The figure shows three views and two pictorial views of one solid part (mm, origin at its lowest corner). Answer the questions. Give positions to 0.01 mm unless a question says otherwise; leave off trailing zeros. Write each loop counter-clockwise with the first axis right and the second up, starting at its lowest first coordinate (ties: lowest second). Pieces come first, ordered by that corner, then holes. Notation, with made-up numbers: (1.5, 70) -> (60.5, 70) arc R30 ccw to (60.5, 102) -> close; hole circle Ø10 at (37.5, -28). An arc over 180 degrees is marked (long way). Use a Markdown table: item, result.
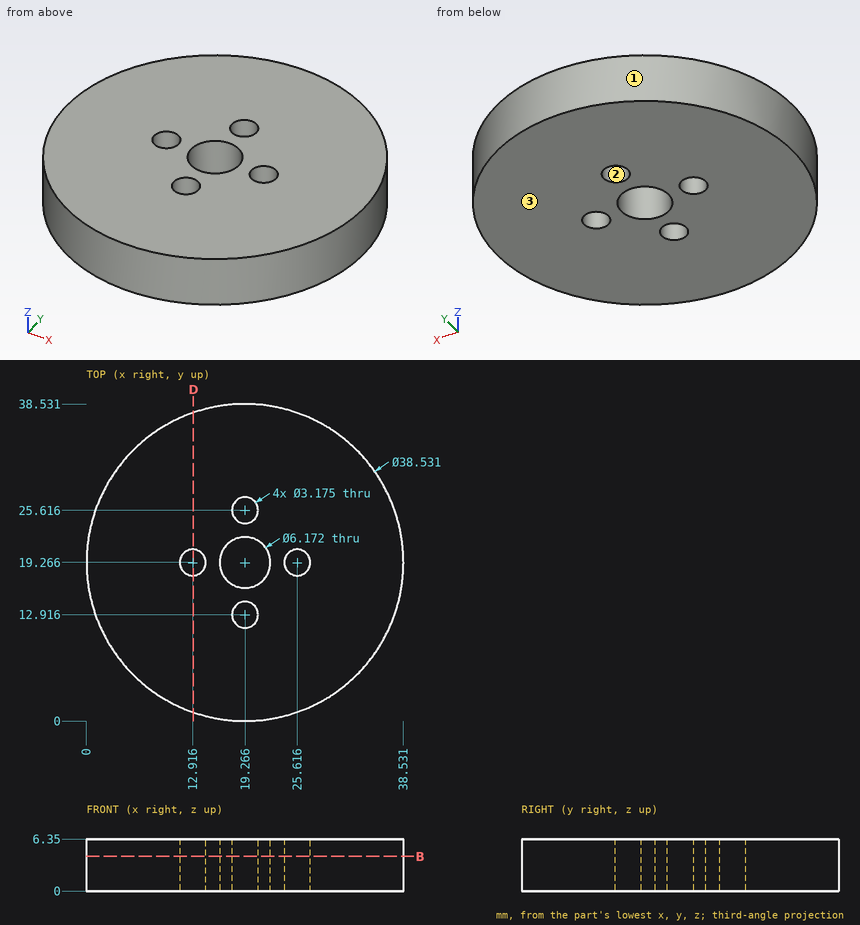
Item 1: A cutting plane is placed at D-D (x = 13). Give the vertices of the cut face in (y, z).
Return value:
| item | result |
|---|---|
| outline | (1.05, 0) -> (17.68, 0) -> (17.68, 6.35) -> (1.05, 6.35) -> close; (20.85, 0) -> (37.48, 0) -> (37.48, 6.35) -> (20.85, 6.35) -> close |
Item 2: Straight lines are drawn through the part: line 1 along X through (y, z) = (19.5, 5.5) (1 decimal); line 2 along X through (y, z) = (19, 1); line 3 along Y through (x, z) = (26, 2) (1 decimal). For each, find the intervals that lie inside material, in ascending order. Write a range as [from, to].
Return value:
| item | result |
|---|---|
| line 1 | [0, 11.3], [14.5, 16.2], [22.3, 24], [27.2, 38.5] |
| line 2 | [0, 11.35], [14.48, 16.19], [22.34, 24.05], [27.18, 38.53] |
| line 3 | [1.2, 17.7], [20.8, 37.3] |
Item 3: For a pull along Y with two mould halves and no side action, classify the marked faces 1, 2 and 3 as +Y half, -Y half, draft (parallel to the pull), parting line (faces both ways), or undercut.
Return value:
| item | result |
|---|---|
| face 1 | parting line |
| face 2 | undercut |
| face 3 | draft |
Item 4: A cutting plane is placed at B-B (z = 4.25). Give the vertices of the cut face in (x, y) (1 decimal).
Return value:
| item | result |
|---|---|
| outline | circle Ø38.5 at (19.3, 19.3); hole circle Ø3.2 at (12.9, 19.3); hole circle Ø6.2 at (19.3, 19.3); hole circle Ø3.2 at (19.3, 12.9); hole circle Ø3.2 at (19.3, 25.6); hole circle Ø3.2 at (25.6, 19.3) |
Item 5: Each of these flat-tipped pins is pushed along its axis until it touches: P1, Ø3, axis at x = 25.62, y = 19.27, coming from the +Z side; P2, Ø2, axis at y = 12.5, z = 2.5, coming from the +X side. Where does it stop, or does it pass through?
Return value:
| item | result |
|---|---|
| P1 | through |
| P2 | x = 37.65 |
